```python
from build123d import *

# Parameters (mm, degrees)
CROQUIS1_R                 = 3.25
SALIENTE_EXTRUIR1_DEPTH    = 30
REDONDEO1_R                = 10
CORTAR_EXTRUIR1_DEPTH      = 46.124827032
CROQUIS3_W                 = 19.168620823
CROQUIS3_H                 = 82.221468015
CORTAR_EXTRUIR2_DEPTH      = 46.124827032
CORTAR_EXTRUIR7_DEPTH      = 44.68352107
CORTAR_EXTRUIR7_DEPTH_BACK = 44.68352107
CROQUIS4_W                 = 3.2
CROQUIS4_H                 = 2.3
REDONDEO2_R                = 1.2
REDONDEO4_R                = 1
CHAMFER1_SIZE              = 0.5
CHAMFER2_SIZE              = 1


with BuildPart() as part:
    # Croquis1 → Saliente-Extruir1 (new body)
    with BuildSketch(Plane.XY):
        with BuildLine():
            Line((-4, 17.433827309), (-8.98691391, 20.296314259))
            ThreePointArc((-8.98691391, 20.296314259), (-9.006535925, 30.69237342), (0, 25.5))
            Line((0, 25.5), (0, -25.5))
            ThreePointArc((0, -25.5), (-9.006535925, -30.69237342), (-8.98691391, -20.296314259))
            Line((-8.98691391, -20.296314259), (-4, -17.433827309))
            Line((-4, -17.433827309), (-4, 17.433827309))
        make_face()
        with Locations((-6, 25.5)):
            Circle(CROQUIS1_R, mode=Mode.SUBTRACT)
        with Locations(Location((-6, -25.5, 0), (0, 0, 180))):
            Circle(CROQUIS1_R, mode=Mode.SUBTRACT)
    extrude(amount=-SALIENTE_EXTRUIR1_DEPTH)

    # Redondeo1
    redondeo1_edges = [part.edges().sort_by_distance(p)[0] for p in [
        (-4, -17.433827309, -15),
        (-4, 17.433827309, -15),
    ]]
    fillet(redondeo1_edges, radius=REDONDEO1_R)

    # Croquis2 → Cortar-Extruir1 (cut, through all)
    with BuildSketch(Plane(origin=(0, 0, 0), x_dir=(0, 0, -1), z_dir=(1, 0, 0))):
        with BuildLine():
            Line((11, 22), (19, 22))
            ThreePointArc((19, 22), (21, 20), (19, 18))
            Line((19, 18), (11, 18))
            ThreePointArc((11, 18), (9, 20), (11, 22))
        make_face()
        with BuildLine():
            Line((11, -22), (19, -22))
            ThreePointArc((19, -22), (21, -20), (19, -18))
            Line((19, -18), (11, -18))
            ThreePointArc((11, -18), (9, -20), (11, -22))
        make_face()
    extrude(amount=-CORTAR_EXTRUIR1_DEPTH, mode=Mode.SUBTRACT)

    # Croquis3 → Cortar-Extruir2 (cut, through all)
    with BuildSketch(Plane(origin=(0, 0, -30), x_dir=(-1, 0, 0), z_dir=(0, 0, -1))):
        with Locations((15.792539244, 3.658464898)):
            Rectangle(CROQUIS3_W, CROQUIS3_H)
    extrude(amount=-CORTAR_EXTRUIR2_DEPTH, mode=Mode.SUBTRACT)

    # Croquis4 → Cortar-Extruir7 (cut, two sides: drawn at the far end of the back side and taken through both)
    with BuildSketch(Plane.ZY.offset(4).offset(-CORTAR_EXTRUIR7_DEPTH_BACK)):
        with Locations((-4.6, 31.35)):
            Rectangle(CROQUIS4_W, CROQUIS4_H)
        with Locations((-25.4, 31.35)):
            Rectangle(CROQUIS4_W, CROQUIS4_H)
        with Locations((-25.4, 19.65)):
            Rectangle(CROQUIS4_W, CROQUIS4_H)
        with Locations((-4.6, 19.65)):
            Rectangle(CROQUIS4_W, CROQUIS4_H)
        with Locations((-4.6, -19.65)):
            Rectangle(CROQUIS4_W, CROQUIS4_H)
        with Locations((-25.4, -19.65)):
            Rectangle(CROQUIS4_W, CROQUIS4_H)
        with Locations((-4.6, -31.35)):
            Rectangle(CROQUIS4_W, CROQUIS4_H)
        with Locations((-25.4, -31.35)):
            Rectangle(CROQUIS4_W, CROQUIS4_H)
    extrude(amount=CORTAR_EXTRUIR7_DEPTH + CORTAR_EXTRUIR7_DEPTH_BACK, mode=Mode.SUBTRACT)

    # Redondeo2
    # the kernel refuses this fillet: 1.2 mm, written as the material it takes off along each edge
    with BuildSketch(Plane(origin=(-6.208228832, 31.496385641, -6.633505757), x_dir=(0.9962436341156765, -0.08659458114680287, 0), z_dir=(0, 0, 1)), Plane(origin=(-6.208228832, 31.496385641, -33.633505757), x_dir=(0.9962436341156765, -0.08659458114680287, 0), z_dir=(0, 0, 1))) as redondeo2_piece_1:
        with BuildLine():
            CenterArc((1.308062073, -1.191165907), REDONDEO2_R, 83.043435968, 101.924289818)
            Line((0.112569712, -1.295079404), (0, 0))
            ThreePointArc((0, 0), (0.726701151, 0.044170466), (1.453402303, 0))
        make_face()
    extrude(amount=10.267011514, mode=Mode.SUBTRACT)
    with BuildSketch(Plane(origin=(-6.208228832, -31.496385641, -33.633505757), x_dir=(0.9962436341156764, 0.08659458114680295, 0), z_dir=(0, 0, 1)), Plane(origin=(-6.208228832, -31.496385641, -6.633505757), x_dir=(0.9962436341156764, 0.08659458114680295, 0), z_dir=(0, 0, 1))) as redondeo2_piece_2:
        with BuildLine():
            CenterArc((1.308062073, 1.191165907), REDONDEO2_R, 175.032274214, 101.924289818)
            Line((0.112569712, 1.295079404), (0, 0))
            ThreePointArc((0, 0), (0.726701151, -0.044170466), (1.453402303, 0))
        make_face()
    extrude(amount=10.267011514, mode=Mode.SUBTRACT)
    with BuildSketch(Plane(origin=(-6.208228832, 28.743322487, -32.736879913), x_dir=(0, 1, 0), z_dir=(0, 0, 1))) as redondeo2_piece_3:
        with BuildLine():
            CenterArc((1.094751965, -1.2), REDONDEO2_R, 90, 77.122346342)
            ThreePointArc((-0.075065865, -0.93255609), (-0.003800627, -0.468993318), (0, 0))
            Line((0, 0), (1.094751965, 0))
        make_face()
    extrude(amount=35.473759826, mode=Mode.SUBTRACT)
    with BuildSketch(Plane(origin=(-6.208228832, 22.256677513, -32.736879913), x_dir=(0, -1, 0), z_dir=(0, 0, 1)), Plane(origin=(-6.208228832, -28.743322487, -32.736879913), x_dir=(0, -1, 0), z_dir=(0, 0, 1))) as redondeo2_piece_4:
        with BuildLine():
            CenterArc((1.094751965, 1.2), REDONDEO2_R, 192.877653658, 77.122346342)
            ThreePointArc((-0.075065865, 0.93255609), (-0.003800627, 0.468993318), (0, 0))
            Line((0, 0), (1.094751965, 0))
        make_face()
    extrude(amount=35.473759826, mode=Mode.SUBTRACT)
    with BuildSketch(Plane(origin=(-6.208228832, 17.911631675, 1.023475891), x_dir=(0.6116158089577609, -0.7911549167090751, 0), z_dir=(0, 0, -1))) as redondeo2_piece_5:
        with BuildLine():
            CenterArc((0.410047777, -1.199775514), REDONDEO2_R, 91.108276989, 36.598151405)
            Line((-0.323891193, -0.250389614), (0, 0))
            ThreePointArc((0, 0), (0.193418763, -0.001870716), (0.386837526, 0))
        make_face()
    extrude(amount=32.046951782, mode=Mode.SUBTRACT)
    with BuildSketch(Plane(origin=(-6.208228832, -22.256677513, -32.736879913), x_dir=(0.9967759569904702, -0.0802352264640189, 0), z_dir=(0, 0, 1))) as redondeo2_piece_6:
        with BuildLine():
            CenterArc((1.108293477, 1.187504709), REDONDEO2_R, 184.602086684, 77.122346342)
            Line((-0.087837672, 1.091222438), (0, 0))
            ThreePointArc((0, 0), (0.467786208, 0.033841412), (0.935572415, 0))
        make_face()
    extrude(amount=35.473759826, mode=Mode.SUBTRACT)
    with BuildSketch(Plane(origin=(-6.208228832, -17.911631675, 1.023475891), x_dir=(0, -1, 0), z_dir=(0, 0, -1))) as redondeo2_piece_7:
        with BuildLine():
            CenterArc((0.409390356, -1.2), REDONDEO2_R, 90, 36.598151405)
            ThreePointArc((-0.306048411, -0.236595946), (-0.151880046, -0.119777999), (0, 0))
            Line((0, 0), (0.409390356, 0))
        make_face()
    extrude(amount=32.046951782, mode=Mode.SUBTRACT)
    with BuildSketch(Plane(origin=(-6.208228832, 31.496385641, -27.433505757), x_dir=(0.9962436341156765, -0.08659458114680287, 0), z_dir=(0, 0, 1))) as redondeo2_piece_8:
        with BuildLine():
            CenterArc((1.308062073, -1.191165907), REDONDEO2_R, 83.043435968, 101.924289818)
            Line((0.112569712, -1.295079404), (0, 0))
            ThreePointArc((0, 0), (0.726701151, 0.044170466), (1.453402303, 0))
        make_face()
    extrude(amount=24.867011514, mode=Mode.SUBTRACT)
    with BuildSketch(Plane(origin=(-6.208228832, -31.496385641, -27.433505757), x_dir=(0.9962436341156764, 0.08659458114680295, 0), z_dir=(0, 0, 1))) as redondeo2_piece_9:
        with BuildLine():
            CenterArc((1.308062073, 1.191165907), REDONDEO2_R, 175.032274214, 101.924289818)
            Line((0.112569712, 1.295079404), (0, 0))
            ThreePointArc((0, 0), (0.726701151, -0.044170466), (1.453402303, 0))
        make_face()
    extrude(amount=24.867011514, mode=Mode.SUBTRACT)

    # Redondeo4
    redondeo4_edges = [part.edges().sort_by_distance(p)[0] for p in [
        (0, -18.5, -25.4),
        (0, -20.8, -25.4),
        (0, -18.5, -4.6),
        (0, -20.8, -4.6),
        (-2.27038876, 30.2, -4.6),
        (0, 18.5, -25.4),
        (0, 20.8, -25.4),
        (0, 18.5, -4.6),
        (0, 20.8, -4.6),
        (-2.27038876, 30.2, -25.4),
    ]]
    fillet(redondeo4_edges, radius=REDONDEO4_R)

    # Chamfer1
    chamfer1_edges = [part.edges().sort_by_distance(p)[0] for p in [
        (0, 0, -30),
        (-4, 0, 0),
        (-4, 0, -30),
        (-6.208228832, -30.017248777, 0),
        (-6.208228832, -30.017248777, -30),
        (-1.339619985, -29.279002265, 0),
        (-6.208228832, 30.017248777, 0),
        (-2.75, 25.5, 0),
        (-6.208228832, 19.74147379, 0),
        (-4.505694572, 14.783364937, 0),
        (-6.208228832, -19.74147379, 0),
        (-2.75, -25.5, 0),
        (-5.946560515, 29.09005463, 0),
        (-5.946560515, 21.90994537, 0),
        (-5.764029285, 31.128499105, 0),
        (-6.147545484, 17.944249464, 0),
        (-6.147545484, -17.944249464, 0),
        (-5.946560515, -21.90994537, 0),
        (-5.946560515, -29.09005463, 0),
        (-5.764029285, -31.128499105, 0),
        (-1.339619985, -29.279002265, -30),
        (-6.208228832, 30.017248777, -30),
        (-2.75, -25.5, -30),
        (-6.208228832, -19.74147379, -30),
        (-4.505694572, -14.783364937, -30),
        (-6.208228832, 19.74147379, -30),
        (-2.75, 25.5, -30),
        (-5.946560515, 29.09005463, -30),
        (-5.946560515, 21.90994537, -30),
        (-6.147545484, 17.944249464, -30),
        (-6.147545484, -17.944249464, -30),
        (-5.946560515, -21.90994537, -30),
        (-5.946560515, -29.09005463, -30),
        (-5.764029285, -31.128499105, -30),
        (-5.764029285, 31.128499105, -30),
        (-4.505694572, -14.783364937, 0),
        (-4.505694572, 14.783364937, -30),
        (-1.339619985, 29.279002265, -30),
        (0, 0, 0),
        (-1.339619985, 29.279002265, 0),
    ]]
    chamfer(chamfer1_edges, length=CHAMFER1_SIZE)

    # Chamfer2
    chamfer2_edges = [part.edges().sort_by_distance(p)[0] for p in [
        (0, 20, -9),
        (0, 18, -15),
        (0, 20, -21),
        (0, 22, -15),
        (0, -20, -9),
        (0, -22, -15),
        (0, -20, -21),
        (0, -18, -15),
    ]]
    chamfer(chamfer2_edges, length=CHAMFER2_SIZE)


solid = part.part
```
Part model, mm, in its own coordinate system. A direction names the side the tool comes from. Give positions to 0.01 mm unless a question says otherwise; leave off trailing zeros. Write each loop counter-clockwise with the first axis right and the second up, starting at its lowest first coordinate (ties: lowest second). Pieces come first, ordered by that corner, then holes. Notation, with made-up numbers: (44.25, -20.75) -> (50.25, -20.75) arc R22 ccw to (50.25, -13.75) -> close; hole circle Ø2 at (54.25, 10). An arc over 180 degrees is marked (long way). Put each result on its own line as item: value. Start each with the question number.
Item 1: Cut at A-A (y = -20). List the corners of the cut face in (x, z).
Item 2: Pull direction Y, two halves, no side cores. Call faces 4 (the face through (-6.208, -21, -25)), 5 (the face through (-3, 20, -3)), 6 (the face through (-4, 30.2, -25)): pulls with the +Y half, pulls with the -Y half, needs draft (parallel to the pull), parting line crosses it, or undercut.
Item 3: Wall check: L1, parallel to Y at x = -1.25, z = -12; L2, parallel to Z at x = -2.75, y = 20.5; L3, parallel to Y at x = -1, z = -11. Give the ranges that are in metal, low to high. Write a range as [from, to].
Item 4: Which spindle directions (+Z, -Z, +X, -X, +Y, -Y) get a long thin tool onto all of the face, cutting with end or side? Do faces 1 (the face through (-0.8, -20, -21.2)), 2 (the face through (-4, 18.5, -5)), 3 (the face through (-2, 0, 0)). Say none if no direction does.
Item 5: Cut at B-B (y = 4.5). List the corners of the cut face in (x, z).
Item 6: Cut at C-C (z = -12). State how many separate pieces and enclosed holes the cut face has, then the cut area to 3 significant figures.
Item 7: Pin check, flat tips, straight feed: pin 1 Ø1.6 at (x, z) = (-3, -4.5) entering from +Y; pin 2 Ø2.5 at (x, z) = (-4, -4.5) entering from -Y; pin 3 Ø10 at (y, z) = (-4, -14.5) entering from -X. Stop position of each tip, or through.
Answer list:
1. outline: (-6.21, -29.5) -> (-5.71, -30) -> (-0.5, -30) -> (0, -29.5) -> (0, -27) -> (-6.21, -27) -> close; (-6.21, -23.8) -> (0, -23.8) -> (0, -22) -> (-1, -21) -> (-6.21, -21) -> close; (-6.21, -9) -> (-1, -9) -> (0, -8) -> (0, -6.2) -> (-6.21, -6.2) -> close; (-6.21, -3) -> (0, -3) -> (0, -0.5) -> (-0.5, 0) -> (-5.71, 0) -> (-6.21, -0.5) -> close
2. face 4: needs draft
2. face 5: undercut
2. face 6: pulls with the +Y half
3. L1: y = [-29.17, -22], [-18, 18], [22, 29.17]
3. L2: z = [-30, -27], [-23.8, -20.94], [-9.06, -6.2], [-3, 0]
3. L3: y = [-28.82, -22], [-18, 18], [22, 28.82]
4. face 1: +X
4. face 2: +X, -X
4. face 3: +Z, +X, -X, +Y, -Y
5. outline: (-4, -29.5) -> (-3.5, -30) -> (-0.5, -30) -> (0, -29.5) -> (0, -0.5) -> (-0.5, 0) -> (-3.5, 0) -> (-4, -0.5) -> close
6. separate pieces: 3
6. enclosed holes: 0
6. area: 216 mm2
7. pin 1: stops at y = 30.2
7. pin 2: stops at y = -30.2
7. pin 3: stops at x = -4
